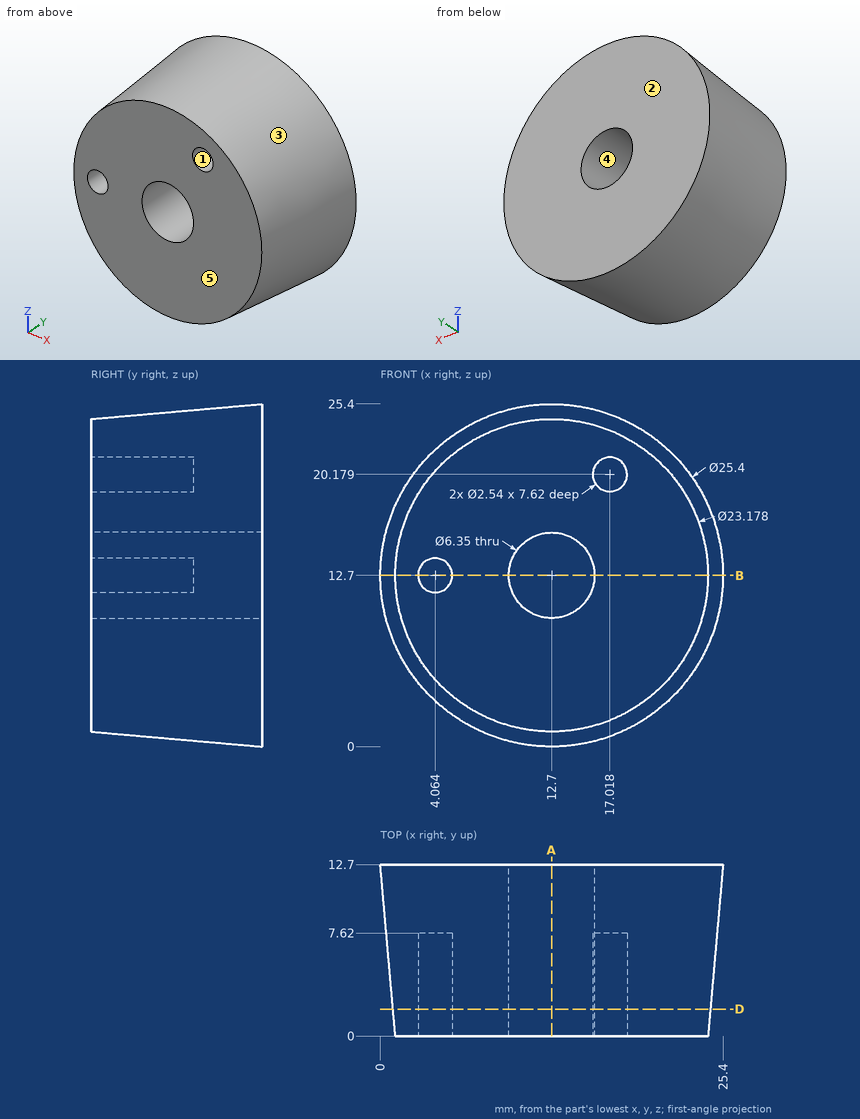
The drawing under review shows one solid part. Ordinate dimensions are in mm from its lowest x, y, z. A direction names the side the tool comes from. Give positions to 0.01 mm unless a question says otherwise; leave off trailing zeros. Loops run counter-clockwise (first coordinate to the right, second up) from the corner with the lowest first, then second, coordinate; pieces in that order, holes last. Notation, with made-up numbers: M 67.5,-32.75 L 78.5,-32.75 A24 cw 78.5,-18.75 Z; hole C 23,-29 d4. An arc over 180 degrees is marked long. One line per question, with ' | ' between items. Start each with the question number.
1. To check wall thickness, follow L1, parallel to X at y = 6, z = 12.7 (1 decimal); L2, parallel to Z at x = 14.25, y = 4.75; L3, parallel to X at y = 11, z = 13.25. State the ranges of each line that lie inside material, in increasing order.
2. Insertion check: P1, Ø0.8, axis at x = 16.5, z = 20, coming from the -Y side; P2, Ø4, axis at x = 22, y = 8.5, coming from the -Z side; P3, Ø5, axis at x = 18.5, y = 9, coming from the -Z side. Each pin has a flat end and moves straight along its axis. Give the tip position at first contact, or say it passes through.
3. Add section D-D (y = 2). Give the number of separate pieces and of enclosed holes in the cut face, plus the area to 3 significant figures.
4. The part is to be moulded in two halves that separate along X. For the marked faces 3, 4 and 5, say which applies: released by +X, released by -X, zero draft, split by the parting line, or undercut.
5. For the marked faces 1 and 2, list the 3-axis set-ups (+Z, -Z, +X, -X, +Y, -Y) from which the entire face can be reached by the end or side of a thin tool; tool diameter is ignored.
6. Add section A-A (x = 12.7). Write out the cut boundary in (y, z) (1 decimal).
7. Add section B-B (z = 12.7). Write out the cut boundary in (x, y) (1 decimal).
Worked out:
1) L1: x = 0.6 to 2.8, 5.3 to 9.5, 15.9 to 24.8 | L2: z = 0.8 to 9.93, 15.47 to 24.6 | L3: x = 0.16 to 9.57, 15.83 to 25.24
2) P1: stops at y = 7.62 | P2: stops at z = 2.74 | P3: stops at z = 0.74
3) separate pieces: 1 | enclosed holes: 3 | area: 393 mm²
4) face 3: split by the parting line | face 4: undercut | face 5: zero draft
5) face 1: -Y | face 2: +Z, -Z, +X, -X, +Y
6) outline: M 0,1.1 L 12.7,0 L 12.7,9.5 L 0,9.5 Z; M 0,15.9 L 12.7,15.9 L 12.7,25.4 L 0,24.3 Z
7) outline: M 0,12.7 L 1.1,0 L 2.8,0 L 2.8,7.6 L 5.3,7.6 L 5.3,0 L 9.5,0 L 9.5,12.7 Z; M 15.9,0 L 24.3,0 L 25.4,12.7 L 15.9,12.7 Z
